Geometry: final body of the model. Coordinates: model frame, mm. A direction names the side the tool comes from. Give positions to 0.01 mm unless a question says otherwise; leave off trailing zeros. Loops run counter-clockwise (first coordinate to the right, second up) from the corner with the lowest first, then second, coordinate; pieces in that order, holes last. Notation, with made-up numbers: (-20.5, 43.5) - (28.5, 43.5) arc R8 cw to (28.5, 51.5) - close; hole circle Ø4 at (62.5, -10.5). An arc over 180 degrees is marked (long way). Use one line per item in the form item = value.
```python
from build123d import *

# Parameters (mm, degrees)
F2_W             = 2000
F2_H             = 1000
F3_DEPTH         = 25
F4_W             = 100
F4_H             = 100
F5_DEPTH         = 700
F5_COPIES2_COUNT = 2
F6_R             = 25
F7_DEPTH         = 100
F7_COPIES2_COUNT = 2
F7_COPIES2_PITCH = 2102.379604


# Not quite as in the source:
# - a pattern or mirror of a feature is missing from the dataset's text; its kind, count and spacing are read off the source's solid


with BuildPart() as f3:
    # F2 (on Top) → F3 (new body)
    with BuildSketch(Plane.XY):
        Rectangle(F2_W, F2_H)
    extrude(amount=F3_DEPTH)

    # F4 (on face) → F5 (join)
    with BuildSketch(Plane.XY.offset(25)):
        with Locations((-950, 450)):
            Rectangle(F4_W, F4_H)
    f5 = extrude(amount=F5_DEPTH)

    # F5_copies: F5 across plane
    add(f5.mirror(Plane(origin=(0, 0, 0), x_dir=(0, 0, 1), z_dir=(1, 0, 0))))

    # F5_copies1: F5 across plane
    add(f5.mirror(Plane(origin=(0, 0, 0), x_dir=(0, 0, -1), z_dir=(0, -1, 0))))

    # F5_copies2: F5 ×2 about axis
    f5_copies2_axis = Axis((0, 0, 0), (0, 0, 1))
    for i in range(1, F5_COPIES2_COUNT):
        add(f5.rotate(f5_copies2_axis, i * 360 / F5_COPIES2_COUNT))

    # F6 (on face) → F7 (cut, through all)
    with BuildSketch(Plane.YZ.offset(-900)):
        with Locations((450, 650)):
            Circle(F6_R)
    f7 = extrude(amount=-F7_DEPTH, mode=Mode.SUBTRACT)

    # F7_copies: F7 across plane
    add(f7.mirror(Plane(origin=(0, 0, 0), x_dir=(0, 0, 1), z_dir=(1, 0, 0))), mode=Mode.SUBTRACT)

    # F7_copies1: F7 across plane
    add(f7.mirror(Plane(origin=(0, 0, 0), x_dir=(0, 0, -1), z_dir=(0, -1, 0))), mode=Mode.SUBTRACT)

    # F7_copies2: F7 ×2
    with Locations(*[Vector(0.9037378389, -0.4280863447, 0) * (i * F7_COPIES2_PITCH) for i in range(1, F7_COPIES2_COUNT)]):
        add(f7, mode=Mode.SUBTRACT)


solid = f3.part
```
(1) Pin query (flat end, axial travel): P1, Ø2, axis at x = 186.5, y = 164.5, coming from the +Z side. Return the tip coordinate at first contact, or that it passes through.
Solution:
P1 = 25
(2) Access query for faces 4 (the face through (900, -449, 370)), 5 (the face through (-14, 7, 0)), 6 (the face through (951, 400, 370)). Directions: +Z, -Z, +X, -X, +Y, -Y. A direction counts if a zero-diameter tool reaches every point of the face in a straight line with its end or side. Return the directions, or none.
Solution:
face_4 = +Z, +Y, -Y
face_5 = -Z, +X, -X, +Y, -Y
face_6 = +Z, +X, -X
(3) Cut plane A-A (z = 650). Give the number of separate pieces and of enclosed holes in the cut face, plus the area to 3 significant figures.
Solution:
separate_pieces = 8
enclosed_holes = 0
area = 20,000 mm2
(4) Pull-direction query (Z, two-part tool) for faces 1 (the face through (-1000, -35, 12)), 2 (the face through (949.3, 461.5, 627.8)), 3 (the face through (-951, 451, 725)); classes: released by +Z, released by -Z, zero draft, split by the parting line, or undercut.
Solution:
face_1 = zero draft
face_2 = undercut
face_3 = released by +Z
(5) Cut plane C-C (y = -450). Return the cut outline in (x, z).
Solution:
outline = (-1000, 0) - (1000, 0) - (1000, 625) - (900, 625) - (900, 25) - (-900, 25) - (-900, 625) - (-1000, 625) - close; (-1000, 675) - (-900, 675) - (-900, 725) - (-1000, 725) - close; (900, 675) - (1000, 675) - (1000, 725) - (900, 725) - close
(6) Material intervals for L1, parallel to X at y = -448.5, z = 396; L2, parallel to Z at x = -963, y = -450; L3, parallel to Z at x = -452.5, y = -449, sorted ascending. Write a range as from..to.
Solution:
L1 = -1000..-900, 900..1000
L2 = 0..625, 675..725
L3 = 0..25
(7) Cut plane D-D (x = 438). Return the cut outline in (y, z), plus the area to 3 significant figures.
Solution:
outline = (-500, 0) - (500, 0) - (500, 25) - (-500, 25) - close
area = 25,000 mm2
(8) Cut plane B-B (z = 292.5). Return the cut outline in (x, y).
Solution:
outline = (-1000, -500) - (-900, -500) - (-900, -400) - (-1000, -400) - close; (-1000, 400) - (-900, 400) - (-900, 500) - (-1000, 500) - close; (900, -500) - (1000, -500) - (1000, -400) - (900, -400) - close; (900, 400) - (1000, 400) - (1000, 500) - (900, 500) - close
